```python
from build123d import *

# Parameters (mm, degrees)
ESQUISSE1_W             = 22.86
ESQUISSE1_H             = 20.32
BOSS_EXTRU_1_DEPTH      = 1.6
ESQUISSE2_R             = 0.45
ENL_V_MAT_EXTRU_1_DEPTH = 26.387611646
D_GAGEMENT_M31_D        = 3.4


with BuildPart() as part:
    # Esquisse1 → Boss.-Extru.1 (new body)
    with BuildSketch(Plane(origin=(0, 0, 0), x_dir=(1, 0, 0), z_dir=(0, 1, 0))):
        with Locations((7.545294118, -6.630147059)):
            Rectangle(ESQUISSE1_W, ESQUISSE1_H)
    extrude(amount=BOSS_EXTRU_1_DEPTH)

    # Esquisse2 → Enlèv. mat.-Extru.1 (cut, through all)
    with BuildSketch(Plane(origin=(0, 1.6, 0), x_dir=(1, 0, 0), z_dir=(0, 1, 0))):
        with Locations((-3.884705882, 3.529852941)):
            Circle(ESQUISSE2_R)
        with Locations((-1.344705882, 3.529852941)):
            Circle(ESQUISSE2_R)
        with Locations((1.195294118, 3.529852941)):
            Circle(ESQUISSE2_R)
        with Locations((3.735294118, 3.529852941)):
            Circle(ESQUISSE2_R)
        with Locations(Location((-1.344705882, 0.989852941, 0), (0, 0, 270))):
            Circle(ESQUISSE2_R)
        with Locations(Location((1.195294118, 0.989852941, 0), (0, 0, 270))):
            Circle(ESQUISSE2_R)
        with Locations(Location((3.735294118, 0.989852941, 0), (0, 0, 270))):
            Circle(ESQUISSE2_R)
        with Locations(Location((-1.344705882, -1.550147059, 0), (0, 0, 270))):
            Circle(ESQUISSE2_R)
        with Locations(Location((1.195294118, -1.550147059, 0), (0, 0, 270))):
            Circle(ESQUISSE2_R)
        with Locations(Location((3.735294118, -1.550147059, 0), (0, 0, 270))):
            Circle(ESQUISSE2_R)
        with Locations(Location((-1.344705882, -4.090147059, 0), (0, 0, 270))):
            Circle(ESQUISSE2_R)
        with Locations(Location((1.195294118, -4.090147059, 0), (0, 0, 270))):
            Circle(ESQUISSE2_R)
        with Locations(Location((3.735294118, -4.090147059, 0), (0, 0, 270))):
            Circle(ESQUISSE2_R)
        with Locations(Location((-1.344705882, -6.630147059, 0), (0, 0, 270))):
            Circle(ESQUISSE2_R)
        with Locations(Location((1.195294118, -6.630147059, 0), (0, 0, 270))):
            Circle(ESQUISSE2_R)
        with Locations(Location((3.735294118, -6.630147059, 0), (0, 0, 270))):
            Circle(ESQUISSE2_R)
        with Locations(Location((-1.344705882, -9.170147059, 0), (0, 0, 270))):
            Circle(ESQUISSE2_R)
        with Locations(Location((1.195294118, -9.170147059, 0), (0, 0, 270))):
            Circle(ESQUISSE2_R)
        with Locations(Location((3.735294118, -9.170147059, 0), (0, 0, 270))):
            Circle(ESQUISSE2_R)
        with Locations(Location((-1.344705882, -11.710147059, 0), (0, 0, 270))):
            Circle(ESQUISSE2_R)
        with Locations(Location((1.195294118, -11.710147059, 0), (0, 0, 270))):
            Circle(ESQUISSE2_R)
        with Locations(Location((3.735294118, -11.710147059, 0), (0, 0, 270))):
            Circle(ESQUISSE2_R)
        with Locations(Location((-1.344705882, -14.250147059, 0), (0, 0, 270))):
            Circle(ESQUISSE2_R)
        with Locations(Location((1.195294118, -14.250147059, 0), (0, 0, 270))):
            Circle(ESQUISSE2_R)
        with Locations(Location((3.735294118, -14.250147059, 0), (0, 0, 270))):
            Circle(ESQUISSE2_R)
        with Locations((-3.884705882, 0.989852941)):
            Circle(ESQUISSE2_R)
        with Locations((-3.884705882, -1.550147059)):
            Circle(ESQUISSE2_R)
        with Locations((-3.884705882, -4.090147059)):
            Circle(ESQUISSE2_R)
        with Locations((-3.884705882, -6.630147059)):
            Circle(ESQUISSE2_R)
        with Locations((-3.884705882, -9.170147059)):
            Circle(ESQUISSE2_R)
        with Locations((-3.884705882, -11.710147059)):
            Circle(ESQUISSE2_R)
        with Locations((-3.884705882, -14.250147059)):
            Circle(ESQUISSE2_R)
        with Locations((6.275294118, 3.529852941)):
            Circle(ESQUISSE2_R)
        with Locations(Location((6.275294118, 0.989852941, 0), (0, 0, 270))):
            Circle(ESQUISSE2_R)
        with Locations(Location((6.275294118, -1.550147059, 0), (0, 0, 270))):
            Circle(ESQUISSE2_R)
        with Locations(Location((6.275294118, -4.090147059, 0), (0, 0, 270))):
            Circle(ESQUISSE2_R)
        with Locations(Location((6.275294118, -6.630147059, 0), (0, 0, 270))):
            Circle(ESQUISSE2_R)
        with Locations(Location((6.275294118, -9.170147059, 0), (0, 0, 270))):
            Circle(ESQUISSE2_R)
        with Locations(Location((6.275294118, -11.710147059, 0), (0, 0, 270))):
            Circle(ESQUISSE2_R)
        with Locations(Location((6.275294118, -14.250147059, 0), (0, 0, 270))):
            Circle(ESQUISSE2_R)
        with Locations((-3.884705882, -16.790147059)):
            Circle(ESQUISSE2_R)
        with Locations((-1.344705882, -16.790147059)):
            Circle(ESQUISSE2_R)
        with Locations((1.195294118, -16.790147059)):
            Circle(ESQUISSE2_R)
        with Locations((3.735294118, -16.790147059)):
            Circle(ESQUISSE2_R)
        with Locations((6.275294118, -16.790147059)):
            Circle(ESQUISSE2_R)
        with Locations((8.815294118, 3.529852941)):
            Circle(ESQUISSE2_R)
        with Locations((11.355294118, 3.529852941)):
            Circle(ESQUISSE2_R)
        with Locations((13.895294118, 3.529852941)):
            Circle(ESQUISSE2_R)
        with Locations((16.435294118, 3.529852941)):
            Circle(ESQUISSE2_R)
        with Locations((18.975294118, 3.529852941)):
            Circle(ESQUISSE2_R)
        with Locations(Location((8.815294118, 0.989852941, 0), (0, 0, 270))):
            Circle(ESQUISSE2_R)
        with Locations(Location((11.355294118, 0.989852941, 0), (0, 0, 270))):
            Circle(ESQUISSE2_R)
        with Locations(Location((13.895294118, 0.989852941, 0), (0, 0, 270))):
            Circle(ESQUISSE2_R)
        with Locations(Location((16.435294118, 0.989852941, 0), (0, 0, 270))):
            Circle(ESQUISSE2_R)
        with Locations((18.975294118, 0.989852941)):
            Circle(ESQUISSE2_R)
        with Locations(Location((8.815294118, -1.550147059, 0), (0, 0, 270))):
            Circle(ESQUISSE2_R)
        with Locations(Location((11.355294118, -1.550147059, 0), (0, 0, 270))):
            Circle(ESQUISSE2_R)
        with Locations(Location((13.895294118, -1.550147059, 0), (0, 0, 270))):
            Circle(ESQUISSE2_R)
        with Locations(Location((16.435294118, -1.550147059, 0), (0, 0, 270))):
            Circle(ESQUISSE2_R)
        with Locations((18.975294118, -1.550147059)):
            Circle(ESQUISSE2_R)
        with Locations(Location((8.815294118, -4.090147059, 0), (0, 0, 270))):
            Circle(ESQUISSE2_R)
        with Locations(Location((11.355294118, -4.090147059, 0), (0, 0, 270))):
            Circle(ESQUISSE2_R)
        with Locations(Location((13.895294118, -4.090147059, 0), (0, 0, 270))):
            Circle(ESQUISSE2_R)
        with Locations(Location((16.435294118, -4.090147059, 0), (0, 0, 270))):
            Circle(ESQUISSE2_R)
        with Locations((18.975294118, -4.090147059)):
            Circle(ESQUISSE2_R)
        with Locations(Location((8.815294118, -6.630147059, 0), (0, 0, 270))):
            Circle(ESQUISSE2_R)
        with Locations(Location((11.355294118, -6.630147059, 0), (0, 0, 270))):
            Circle(ESQUISSE2_R)
        with Locations(Location((13.895294118, -6.630147059, 0), (0, 0, 270))):
            Circle(ESQUISSE2_R)
        with Locations(Location((16.435294118, -6.630147059, 0), (0, 0, 270))):
            Circle(ESQUISSE2_R)
        with Locations((18.975294118, -6.630147059)):
            Circle(ESQUISSE2_R)
        with Locations(Location((8.815294118, -9.170147059, 0), (0, 0, 270))):
            Circle(ESQUISSE2_R)
        with Locations(Location((11.355294118, -9.170147059, 0), (0, 0, 270))):
            Circle(ESQUISSE2_R)
        with Locations(Location((13.895294118, -9.170147059, 0), (0, 0, 270))):
            Circle(ESQUISSE2_R)
        with Locations(Location((16.435294118, -9.170147059, 0), (0, 0, 270))):
            Circle(ESQUISSE2_R)
        with Locations((18.975294118, -9.170147059)):
            Circle(ESQUISSE2_R)
        with Locations(Location((8.815294118, -11.710147059, 0), (0, 0, 270))):
            Circle(ESQUISSE2_R)
        with Locations(Location((11.355294118, -11.710147059, 0), (0, 0, 270))):
            Circle(ESQUISSE2_R)
        with Locations(Location((13.895294118, -11.710147059, 0), (0, 0, 270))):
            Circle(ESQUISSE2_R)
        with Locations(Location((16.435294118, -11.710147059, 0), (0, 0, 270))):
            Circle(ESQUISSE2_R)
        with Locations((18.975294118, -11.710147059)):
            Circle(ESQUISSE2_R)
        with Locations(Location((8.815294118, -14.250147059, 0), (0, 0, 270))):
            Circle(ESQUISSE2_R)
        with Locations(Location((11.355294118, -14.250147059, 0), (0, 0, 270))):
            Circle(ESQUISSE2_R)
        with Locations(Location((13.895294118, -14.250147059, 0), (0, 0, 270))):
            Circle(ESQUISSE2_R)
        with Locations(Location((16.435294118, -14.250147059, 0), (0, 0, 270))):
            Circle(ESQUISSE2_R)
        with Locations((18.975294118, -14.250147059)):
            Circle(ESQUISSE2_R)
        with Locations((8.815294118, -16.790147059)):
            Circle(ESQUISSE2_R)
        with Locations((11.355294118, -16.790147059)):
            Circle(ESQUISSE2_R)
        with Locations((13.895294118, -16.790147059)):
            Circle(ESQUISSE2_R)
        with Locations((16.435294118, -16.790147059)):
            Circle(ESQUISSE2_R)
        with Locations((18.975294118, -16.790147059)):
            Circle(ESQUISSE2_R)
    extrude(amount=-ENL_V_MAT_EXTRU_1_DEPTH, mode=Mode.SUBTRACT)

    # Dégagement M31 (through all)
    with Locations(Plane(origin=(0, 1.6, 0), x_dir=(1, 0, 0), z_dir=(0, 1, 0))):
        with Locations((13.895294118, -6.630147059), (1.195294118, -6.630147059)):
            Hole(D_GAGEMENT_M31_D / 2)


solid = part.part
```
Geometry check sheet. Reference: the model listing, model coordinates, mm. Coordinates: 2 decimals unless noted, no trailing zeros. Order: outer loops, then holes, each group sorted by start corner. A loop starts at its lowest first (then second) coordinate and runs counter-clockwise, first axis right, second up.
Item 1: Section check B-B (x = 12.75). Enter the section's corners in (y, z).
Item 2: Mould release check, pull along Z, two halves, no side actions. Record for faces 1 (the cylindrical face through (16.45, 0.81, 16.34)), 2 (the flat face through (18, 1, -3.53)), 3 (the flat face through (7, 0, 6)), 4 (the cylindrical face through (11.8, 0.81, 1.49)): released by +Z, released by -Z, zero draft, split by the parting line, or undercut.
Item 3: Section check A-A (z = 8). Enter the section's corners in (x, y).
Item 4: Section check C-C (y = 1.35). Count the separate pieces of the cut face and the enclosed holes in it, plus the area to 3 significant figures.
Item 5: Scan lines: line 1 along X through (y, z) = (1.2, 5.25); line 2 along X through (y, z) = (0.65, 7.5); line 3 along Z through (x, y) = (15, 1). Record each from-to range of solid material in increasing order.
Check sheet entries:
1. outline: (0, -3.53) - (1.6, -3.53) - (1.6, 5.37) - (0, 5.37) - close; (0, 7.89) - (1.6, 7.89) - (1.6, 16.79) - (0, 16.79) - close
2. face 1: released by +Z
2. face 2: released by -Z
2. face 3: zero draft
2. face 4: undercut
3. outline: (-3.88, 0) - (0.19, 0) - (0.19, 1.6) - (-3.88, 1.6) - close; (2.2, 0) - (12.89, 0) - (12.89, 1.6) - (2.2, 1.6) - close; (14.9, 0) - (18.98, 0) - (18.98, 1.6) - (14.9, 1.6) - close
4. separate pieces: 1
4. enclosed holes: 56
4. area: 402 mm2
5. line 1: x = -3.88 to 0.2, 2.19 to 12.9, 14.89 to 18.98
5. line 2: x = -3.88 to -0.27, 2.66 to 12.43, 15.36 to 18.98
5. line 3: z = -3.53 to 5.34, 7.92 to 16.79
